Could you check a few things on this model? Use its own coordinates, in mm. Give positions to 0.01 mm unless a question says otherwise; leave off trailing zeros. Loops run counter-clockwise (first coordinate to the right, second up) from the corner with the lowest first, then second, coordinate; pieces in that order, holes last.
1. For P1, Ø1.5, axis at y = 11, z = -0.5, coming from the -X side (3 decimals); P2, Ø1.5, axis at x = -447, z = -1.5, coming from the +Y side; P3, Ø3, axis at x = -438.5, y = 9, coming from the -Z side, each with a flat end and sliding along its axis, tell me the tip position at first contact or that it passes through.
2. I need wall thicknesses on line 1 along Z through (x, y) = (-446, 0); line 2 along X through (y, z) = (-6, -16); line 3 along X through (y, z) = (5.5, -1). Which ranges of each line are inside material? Lowest first, please.
3. Thinking about a two-plate mould opening in Z: for faces 1 (the flat face through (-434.342, -9, -8)), 2 (the flat face through (-450, 0, 0)), 3 (the cylindrical face through (-441.184, -1.404, -6.323)), 4 (the cylindrical face through (-445.16, -7.66, -5.87)), which applies, +Z half, -Z half, draft (parallel to the pull), parting line (faces both ways), or undercut?
4. Imagine slicing it at A-A (y = 0). List the corners of the cut face in (x, z) for me, plus the area to 3 significant figures.
5. Imagine slicing it at C-C (x = -439.25). List the corners of the cut face in (y, z) for me.
```python
from build123d import *


with BuildPart() as part:
    # 草图1 → 旋转1 (revolve)
    with BuildSketch(Plane.XY):
        with BuildLine():
            Line((-455, 8.382), (-455, 0))
            Line((-455, 0), (-450, 0))
            Line((-450, 0), (-450, 6.477))
            Line((-450, 6.477), (-432.612413979, 6.477))
            ThreePointArc((-432.612413979, 6.477), (-431.714388367, 6.848974388), (-431.342413979, 7.747))
            Line((-431.342413979, 7.747), (-431.342413979, 18.73))
            ThreePointArc((-431.342413979, 18.73), (-431.714388367, 19.628025612), (-432.612413979, 20))
            Line((-432.612413979, 20), (-433.072413979, 20))
            ThreePointArc((-433.072413979, 20), (-433.970439591, 19.628025612), (-434.342413979, 18.73))
            Line((-434.342413979, 18.73), (-434.342413979, 11.652))
            ThreePointArc((-434.342413979, 11.652), (-434.928200417, 10.237786438), (-436.342413979, 9.652))
            Line((-436.342413979, 9.652), (-453.73, 9.652))
            ThreePointArc((-453.73, 9.652), (-454.628025612, 9.280025612), (-455, 8.382))
        make_face()
    revolve(axis=Axis((-455.001250002, 0, 0), (1, 0, 0)))


solid = part.part
```
Derived:
1. P1: stops at x = -434.905
1. P2: stops at y = 9.62
1. P3: stops at z = -6.08
2. line 1: z = -9.65 to -6.48, 6.48 to 9.65
2. line 2: x = -434.34 to -431.34
2. line 3: x = -455 to -450
3. face 1: draft
3. face 2: undercut
3. face 3: undercut
3. face 4: parting line
4. outline: (-455, -8.38) arc R1.27 ccw to (-453.73, -9.65) - (-436.34, -9.65) arc R2 cw to (-434.34, -11.65) - (-434.34, -18.73) arc R1.27 ccw to (-433.07, -20) - (-432.61, -20) arc R1.27 ccw to (-431.34, -18.73) - (-431.34, -7.75) arc R1.27 ccw to (-432.61, -6.48) - (-450, -6.48) - (-450, 6.48) - (-432.61, 6.48) arc R1.27 ccw to (-431.34, 7.75) - (-431.34, 18.73) arc R1.27 ccw to (-432.61, 20) - (-433.07, 20) arc R1.27 ccw to (-434.34, 18.73) - (-434.34, 11.65) arc R2 cw to (-436.34, 9.65) - (-453.73, 9.65) arc R1.27 ccw to (-455, 8.38) - close
4. area: 276 mm2
5. outline: circle Ø19.3 at (0, 0); hole circle Ø12.95 at (0, 0)
